Read the model definition and answer for the solid it produces. Units are mm, in the model's axes. A direction names the side the tool comes from. Give positions to 0.01 mm unless a question says otherwise; leave off trailing zeros. Order: outer loops, then holes, each group sorted by start corner. A loop starts at its lowest first (then second) coordinate and runs counter-clockwise, first axis right, second up. Notation, with made-up numbers: M 19,65 L 70,65 A9 cw 70,74 Z; hole C -1,18 d4. An arc over 180 degrees is marked long. One line per item, written item: value.
from build123d import *

# Parameters (mm, degrees)
BOSS_EXTRUDE1_DEPTH = 10
SKETCH2_W           = 20
SKETCH2_H           = 14
BOSS_EXTRUDE2_DEPTH = 20
SKETCH3_W           = 20
SKETCH3_H           = 5
BOSS_EXTRUDE3_DEPTH = 20
SKETCH4_R           = 1.5
CUT_EXTRUDE1_DEPTH  = 84.402637848
CIRPATTERN1_COUNT   = 3
SKETCH5_R           = 2.5
CUT_EXTRUDE2_DEPTH  = 117.266161556
SKETCH8_W           = 20
SKETCH8_H           = 14
BOSS_EXTRUDE7_DEPTH = 5
BOSS_EXTRUDE8_DEPTH = 10


with BuildPart() as part:
    # Sketch1 → Boss-Extrude1 (new body)
    with BuildSketch(Plane(origin=(0, 0, 0), x_dir=(1, 0, 0), z_dir=(0, 1, 0))):
        Polygon((0, 0), (-10, 5.773502692), (-10, 80), (10, 80), (10, 5.773502692), align=None)
    boss_extrude1 = extrude(amount=BOSS_EXTRUDE1_DEPTH)

    # Sketch2 → Boss-Extrude2 (add)
    with BuildSketch(Plane(origin=(0, 10, 0), x_dir=(1, 0, 0), z_dir=(0, 1, 0))):
        with Locations((0, 73)):
            Rectangle(SKETCH2_W, SKETCH2_H)
    boss_extrude2 = extrude(amount=BOSS_EXTRUDE2_DEPTH)

    # Sketch3 → Boss-Extrude3 (add)
    with BuildSketch(Plane(origin=(0, 30, 0), x_dir=(1, 0, 0), z_dir=(0, 1, 0))):
        with Locations((0, 77.5)):
            Rectangle(SKETCH3_W, SKETCH3_H)
        with Locations((0, 68.5)):
            Rectangle(SKETCH3_W, SKETCH3_H)
    boss_extrude3 = extrude(amount=BOSS_EXTRUDE3_DEPTH)

    # Sketch4 → Cut-Extrude1 (cut, symmetric)
    with BuildSketch(Plane.XY.offset(-66)):
        with Locations((0, 47)):
            Circle(SKETCH4_R)
    cut_extrude1 = extrude(amount=CUT_EXTRUDE1_DEPTH, both=True, mode=Mode.SUBTRACT)

    # CirPattern1: Boss-Extrude1, Boss-Extrude2, Boss-Extrude3, Cut-Extrude1 ×3 about axis
    cirpattern1_axis = Axis((0, 0, 0), (0, 1, 0))
    add([boss_extrude1.rotate(cirpattern1_axis, i * 360 / CIRPATTERN1_COUNT) for i in range(1, CIRPATTERN1_COUNT)])
    add([boss_extrude2.rotate(cirpattern1_axis, i * 360 / CIRPATTERN1_COUNT) for i in range(1, CIRPATTERN1_COUNT)])
    add([boss_extrude3.rotate(cirpattern1_axis, i * 360 / CIRPATTERN1_COUNT) for i in range(1, CIRPATTERN1_COUNT)])
    add([cut_extrude1.rotate(cirpattern1_axis, i * 360 / CIRPATTERN1_COUNT) for i in range(1, CIRPATTERN1_COUNT)], mode=Mode.SUBTRACT)

    # Sketch5 → Cut-Extrude2 (cut, through all)
    with BuildSketch(Plane(origin=(0, 10, 0), x_dir=(1, 0, 0), z_dir=(0, 1, 0))):
        with Locations(Location((0, 0, 0), (0, 0, 270))):
            Circle(SKETCH5_R)
    extrude(amount=-CUT_EXTRUDE2_DEPTH, mode=Mode.SUBTRACT)

    # Sketch8 → Boss-Extrude7 (add)
    with BuildSketch(Plane(origin=(0, 0, 0), x_dir=(1, 0, 0), z_dir=(0, 1, 0))):
        with Locations((0, 87)):
            Rectangle(SKETCH8_W, SKETCH8_H)
    extrude(amount=BOSS_EXTRUDE7_DEPTH)

    # Sketch11 → Boss-Extrude8 (add)
    with BuildSketch(Plane(origin=(0, 0, 0), x_dir=(1, 0, 0), z_dir=(0, 1, 0))):
        Polygon((-15.5, 94), (15.5, 94), (26, 104.5), (26, 135.5), (15.5, 146), (-15.5, 146), (-26, 135.5), (-26, 104.5), align=None)
    extrude(amount=BOSS_EXTRUDE8_DEPTH)


solid = part.part
1) Find section C-C, the plane y = 13.5. Write down the section's boundary in (x, z).
Reported:
outline: M -74.28,31.34 L -62.16,24.34 L -52.16,41.66 L -64.28,48.66 Z; M -10,-80 L 10,-80 L 10,-66 L -10,-66 Z; M 52.16,41.66 L 62.16,24.34 L 74.28,31.34 L 64.28,48.66 Z
2) Which of the six approach directions +Z, -Z, +X, -X, +Y, -Y give full straight-line access (tool end or side, diameter ignored) to faces 1 (the face through (10, 8, -59)), 2 (the face through (-61.42, 39.86, 35.62)), 3 (the face through (0, 30, -66)), 4 (the face through (0, 30, -73)), 5 (the face through (-45.976, 7.983, 38.091))?
Reported:
face 1: +X, +Y, -Y
face 2: +Y
face 3: +Z, +X, -X, +Y
face 4: +X, -X, +Y
face 5: +Z, +Y, -Y
3) Consider probe 1 along Y at (x, z) = (0, -77); probe 2 along Y at (x, z) = (-43, 26); probe 3 along Z at (x, y) = (6, 44). Determine where each line is inside the solid, lowest interval first.
Reported:
probe 1: y = 0 to 45.5, 48.5 to 50
probe 2: y = 0 to 10
probe 3: z = -80 to -75, -71 to -66
4) Find section B-B, the plane z = 0. Write down the section's boundary in (x, y), plus the area to 3 significant figures.
Reported:
outline: M -20,0 L -2.5,0 L -2.5,10 L -20,10 Z; M 2.5,0 L 20,0 L 20,10 L 2.5,10 Z
area: 350 mm^2
5) Determine the mould class of faces 6 (the face through (-57.1, 29.7, 33.1)), 7 (the face through (-69.212, 24.65, 40.121)), 8 (the face through (55.976, 7.983, 20.771)) for opening direction Z: +Z half, -Z half, draft (parallel to the pull), parting line (faces both ways), or undercut.
Reported:
face 6: -Z half
face 7: +Z half
face 8: undercut
6) Each of these flat-tipped pins is pushed along its axis until it touches: pin 1 Ø6 at (x, y) = (43.5, 11) entering from +Z; pin 2 Ø8 at (y, z) = (7.5, -117) entering from -X; pin 3 Ø22 at (x, y) = (-1.5, 44) entering from +Z; pin 4 Ø11 at (x, z) = (-63, 37) entering from +Y. Where does it stop, or does it pass through?
Reported:
pin 1: stops at z = 38.29
pin 2: stops at x = -26
pin 3: stops at z = -66
pin 4: stops at y = 50
7) Find section A-A, the plane y = 41. Write down the section's boundary in (x, z), plus the area to 3 significant figures.
Reported:
outline: M -74.28,31.34 L -69.95,28.84 L -59.95,46.16 L -64.28,48.66 Z; M -66.49,26.84 L -62.16,24.34 L -52.16,41.66 L -56.49,44.16 Z; M -10,-80 L 10,-80 L 10,-75 L -10,-75 Z; M -10,-71 L 10,-71 L 10,-66 L -10,-66 Z; M 52.16,41.66 L 62.16,24.34 L 66.49,26.84 L 56.49,44.16 Z; M 59.95,46.16 L 69.95,28.84 L 74.28,31.34 L 64.28,48.66 Z
area: 600 mm^2
8) Find section D-D, the plane z = -63. Write down the section's boundary in (x, y), plus the area to 3 significant figures.
Reported:
outline: M -10,0 L 10,0 L 10,10 L -10,10 Z
area: 200 mm^2
